from build123d import *

# Parameters (mm, degrees)
BOSS_EXTRUDE1_DEPTH = 59.999999888
SKETCH2_W           = 25.4
SKETCH2_H           = 12.017000096
SKETCH2_H_2         = 35.282999792
CUT_EXTRUDE1_DEPTH  = 13.7
SKETCH3_R           = 0.877000024
CUT_EXTRUDE2_DEPTH  = 48.982999792
SKETCH4_R           = 3.175
CUT_EXTRUDE3_DEPTH  = 48.982999792
SKETCH5_W           = 50.8
SKETCH5_H           = 4.7625
CUT_EXTRUDE4_DEPTH  = 60.999999888
FILLET1_R           = 2.54


with BuildPart() as part:
    # Sketch1 → Boss-Extrude1 (new body)
    with BuildSketch(Plane(origin=(0, 0, 0), x_dir=(1, 0, 0), z_dir=(0, 1, 0))):
        with BuildLine():
            Line((0, 6.35), (114.3, 6.35))
            ThreePointArc((114.3, 6.35), (120.65, 0), (114.3, -6.35))
            Line((114.3, -6.35), (0, -6.35))
            ThreePointArc((0, -6.35), (-6.35, 0), (0, 6.35))
        make_face()
        with BuildLine():
            Line((118.790128061, 4.490128061), (127.770384182, -4.490128061))
            ThreePointArc((127.770384182, -4.490128061), (127.770384182, -13.470384182), (118.790128061, -13.470384182))
            Line((118.790128061, -13.470384182), (109.809871939, -4.490128061))
            ThreePointArc((109.809871939, -4.490128061), (109.809871939, 4.490128061), (118.790128061, 4.490128061))
        make_face()
    extrude(amount=BOSS_EXTRUDE1_DEPTH)

    # Sketch2 → Cut-Extrude1 (cut, through all)
    with BuildSketch(Plane.XY.offset(6.35)):
        with Locations((6.35, 6.008500048)):
            Rectangle(SKETCH2_W, SKETCH2_H)
        with Locations((6.35, 42.358499992)):
            Rectangle(SKETCH2_W, SKETCH2_H_2)
    extrude(amount=-CUT_EXTRUDE1_DEPTH, mode=Mode.SUBTRACT)

    # Sketch3 → Cut-Extrude2 (cut, through all)
    with BuildSketch(Plane.XZ.offset(-12.017000096)):
        with Locations((6.99999997, 0)):
            Circle(SKETCH3_R)
        with Locations((16.000000004, 0)):
            Circle(SKETCH3_R)
    extrude(amount=-CUT_EXTRUDE2_DEPTH, mode=Mode.SUBTRACT)

    # Sketch4 → Cut-Extrude3 (cut, through all)
    with BuildSketch(Plane.XZ.offset(-12.017000096)):
        Circle(SKETCH4_R)
    extrude(amount=-CUT_EXTRUDE3_DEPTH, mode=Mode.SUBTRACT)

    # Sketch5 → Cut-Extrude4 (cut, through all)
    with BuildSketch(Plane(origin=(0, 59.999999888, 0), x_dir=(1, 0, 0), z_dir=(0, 1, 0))):
        with Locations((48.41875, 0)):
            Rectangle(SKETCH5_W, SKETCH5_H)
        with BuildLine():
            Line((80.16875, 2.38125), (80.16875, -2.38125))
            Line((80.16875, -2.38125), (113.313653955, -2.38125))
            Line((113.313653955, -2.38125), (121.596458098, -10.664054144))
            ThreePointArc((121.596458098, -10.664054144), (124.964054144, -10.664054144), (124.964054144, -7.296458098))
            Line((124.964054144, -7.296458098), (115.983798023, 1.683798023))
            ThreePointArc((115.983798023, 1.683798023), (115.211264923, 2.199988137), (114.3, 2.38125))
            Line((114.3, 2.38125), (80.16875, 2.38125))
        make_face()
    extrude(amount=-CUT_EXTRUDE4_DEPTH, mode=Mode.SUBTRACT)

    # Fillet1
    fillet1_edges = [part.edges().sort_by_distance(p)[0] for p in [
        (116.730039796, 0, -5.866635031),
        (123.280256121, 0, 0),
        (65.359871939, 0, 6.35),
        (66.675, 0, -6.35),
        (19.05, 0, 0),
        (127.770384182, 0, 13.470384182),
        (115.22993597, 0, 9.910192091),
    ]]
    fillet(fillet1_edges, radius=FILLET1_R)


solid = part.part
The model under review builds one solid part; all positions refer to its coordinate system, in mm. A direction names the side the tool comes from. Round coordinates to 2 decimals unless told otherwise and drop trailing zeros. Loops run counter-clockwise (first coordinate to the right, second up) from the corner with the lowest first, then second, coordinate; pieces in that order, holes last. Notation, with made-up numbers: M 64.25,-33 L 68.25,-33 A11 cw 68.25,-16 Z; hole C 16,24.25 d11. An arc over 180 degrees is marked long. Answer as CSV lines item,"result". Start each with the question number.
Item 1: Insertion check: P1, Ø8.5, axis at x = 0, z = 0, coming from the +Y side; P2, Ø17, axis at x = 74.5, y = 39, coming from the +Z side; P3, Ø4.5, axis at y = 8, z = -0.5, coming from the -X side. Each pin has a flat end and moves straight along its axis. Give the tip position at first contact, or say it passes through.
Item 2: Consider section A-A (y = 18). State how many separate pieces and enclosed holes the cut face has, then the cut area to 3 significant figures.
Item 3: Wall thickness on line 1 (Z direction, x = 97, y = 15); line 2 (X direction, y = 10.5, z = 1.5); line 3 (X direction, y = 43, z = 0.5): over which ranges is each line inside the solid? List them lowest first. Write a range as [from, to].
Item 4: For faces 1 (the face through (9, 24.717, 0)), 2 (the face through (23.019, 30, 0)), 3 (the face through (19.05, 7, 0)), list the 3-axis set-ups (+Z, -Z, +X, -X, +Y, -Y) from which the entire face can be reached by the end or side of a thin tool; tool diameter is ignored.
Item 5: Consider section D-D (x = 11). Write out the cut boundary in (y, z), then the cut area to 3 significant figures.
Item 6: Consider section B-B (x = 44). Write out the cut boundary in (y, z), then the cut area to 3 significant figures.
Item 7: Consider section C-C (y = 27.5). Write out the cut boundary in (x, z), then the cut area to 3 significant figures.
Item 8: Mouldability with a two-part tool opening along X and no side actions: class faces 4 (the face through (115.28, 30.87, 9.96)), 5 (the face through (127.87, 30.87, 13.37)), 6 (the face through (48, 30, -2.381)) as released by +X, released by -X, zero draft, split by the parting line, or undercut.
Answer:
1,P1,"stops at y = 24.72"
1,P2,"stops at z = 6.35"
1,P3,"stops at x = 19.05"
2,separate pieces,"1"
2,enclosed holes,"5"
2,area,"1,230 mm^2"
3,line 1,"z = [-6.35, -2.38], [2.38, 6.35]"
3,line 2,"x = [19.05, 23.02], [73.82, 80.17], [119.17, 124.78]"
3,line 3,"x = [19.05, 23.02], [73.82, 80.17], [118.17, 123.78]"
4,face 1,"+Z, -Z, -X, +Y"
4,face 2,"+Y, -Y"
4,face 3,"+Z, -Z, -X, -Y"
5,outline,"M 12.02,-6.35 L 24.72,-6.35 L 24.72,6.35 L 12.02,6.35 Z"
5,area,"161 mm^2"
6,outline,"M 0,-3.81 A2.54 ccw 2.54,-6.35 L 60,-6.35 L 60,-2.38 L 0,-2.38 Z; M 0,2.38 L 60,2.38 L 60,6.35 L 2.54,6.35 A2.54 ccw 0,3.81 Z"
6,area,"473 mm^2"
7,outline,"M 19.05,-6.35 L 114.3,-6.35 A6.35 ccw 118.79,-4.49 L 127.77,4.49 A6.35 ccw 118.79,13.47 L 111.67,6.35 L 19.05,6.35 Z; hole M 23.02,-2.38 L 73.82,-2.38 L 73.82,2.38 L 23.02,2.38 Z; hole M 80.17,-2.38 L 114.3,-2.38 A2.38 ccw 115.98,-1.68 L 124.96,7.3 A2.38 ccw 121.6,10.66 L 113.31,2.38 L 80.17,2.38 Z"
7,area,"960 mm^2"
8,face 4,"released by -X"
8,face 5,"split by the parting line"
8,face 6,"undercut"
